The figure shows three views and two pictorial views of one solid part (mm, origin at its lowest corner). Answer the questions. A direction names the side the tool comes from. Round coordinates to 2 decimals unless told otherwise and drop trailing zeros. Order: outer loops, then holes, each group sorted by start corner. A loop starts at its lowest first (then second) coordinate and runs counter-clockwise, first axis right, second up. Notation, with made-up numbers: (-38, -10) -> (15, -10) arc R22 cw to (15, -2) -> close; hole circle Ø5 at (4.5, 85). An arc over 180 degrees is marked (long way). Answer as a JSON object with one key per item and string values. Group by question number.
Item 1: Section A-A, the plane x = 25 is taken. Write down the section's boundary in (y, z).
Item 2: Section C-C, the plane z = 25 is taken. Write down the section's boundary in (x, y).
Item 3: Given P1, Ø10, axis at y = 10, z = 26.5, coming from the -X side; P2, Ø2, axis at y = 13.5, z = 37, coming from the -X side; P3, Ø4, axis at x = 25, y = 10, coming from the +Z side; P4, Ø3, axis at x = 43, y = 17.5, coming from the -Z side (3 decimals), each flat-ended and moving along its own axis, determine where each tip first touches the part or whether it passes through.
Item 4: Section B-B, the plane y = 27 is taken. Count the separate pieces of the cut face and the enclosed holes in it.
Item 5: The mould has two halves that part along X. Classify the marked faces 5, 6 and 7: pulls with the +X half, pulls with the -X half, needs draft (parallel to the pull), parting line crosses it, or undercut.
Item 6: For the marked faces 1, 2, 3 and 4, determine the directions among +Z, -Z, +X, -X, +Y, -Y from which every point of the face is accessible in a straight line to the end or side of a thin tool.
Item 7: Consider probe 1 along X at (y, z) = (26, 8) (1 decimal); probe 2 along Y at (x, z) = (8.5, 22.5). Determine where each line is inside the solid, lowest interval first. Write a range as from..to.
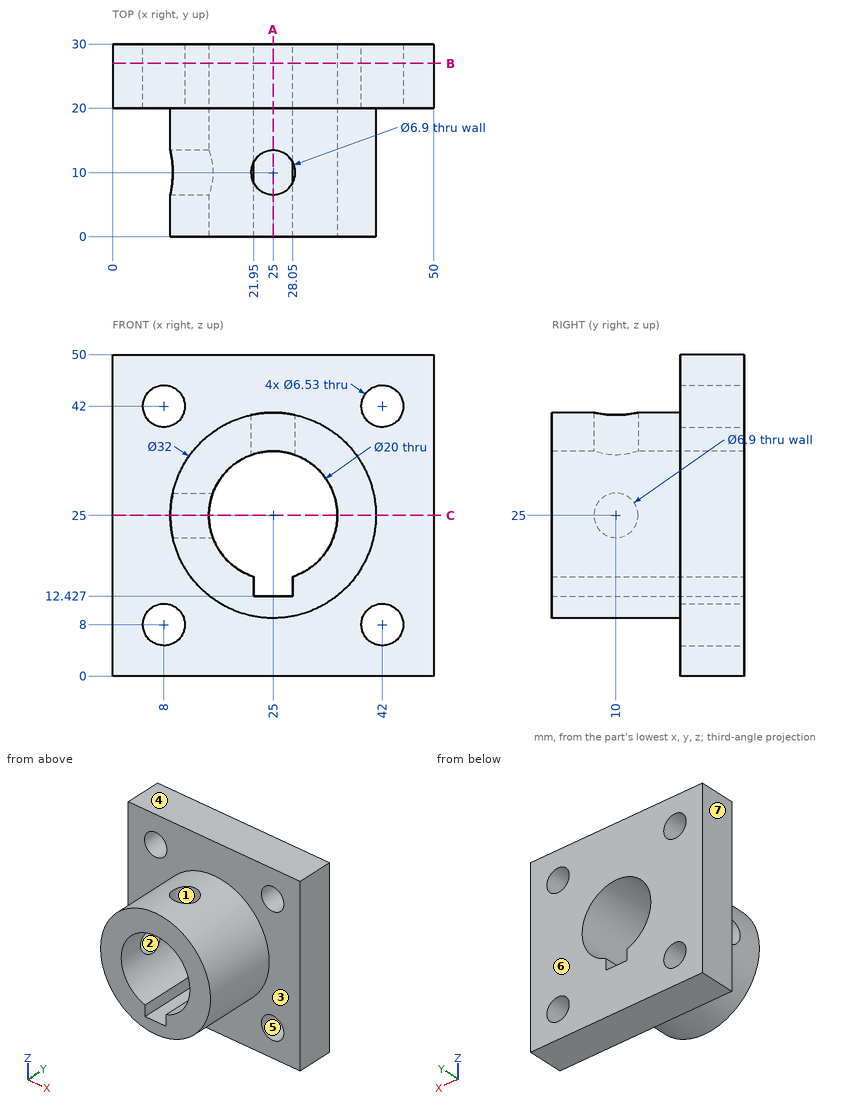
Values found:
{
 "1": {"outline": "(0, 9) -> (20, 9) -> (20, 0) -> (30, 0) -> (30, 12.43) -> (0, 12.43) -> close; (0, 35) -> (6.55, 35) -> (6.55, 41) -> (0, 41) -> close; (13.45, 35) -> (30, 35) -> (30, 50) -> (20, 50) -> (20, 41) -> (13.45, 41) -> close"},
 "2": {"outline": "(0, 20) -> (9, 20) -> (9, 13.45) -> (15, 13.45) -> (15, 30) -> (0, 30) -> close; (9, 0) -> (15, 0) -> (15, 6.55) -> (9, 6.55) -> close; (35, 0) -> (41, 0) -> (41, 20) -> (50, 20) -> (50, 30) -> (35, 30) -> close"},
 "3": {"P1": "x = 9", "P2": "x = 13.38", "P3": "z = 12.43", "P4": "through"},
 "4": {"separate pieces": "1", "enclosed holes": "5"},
 "5": {"face 5": "undercut", "face 6": "needs draft", "face 7": "pulls with the -X half"},
 "6": {"face 1": "+Z", "face 2": "-X", "face 3": "-Y", "face 4": "+Z, +X, -X, +Y, -Y"},
 "7": {"probe 1": "0..4.7, 11.3..38.7, 45.3..50", "probe 2": "20..30"}
}
